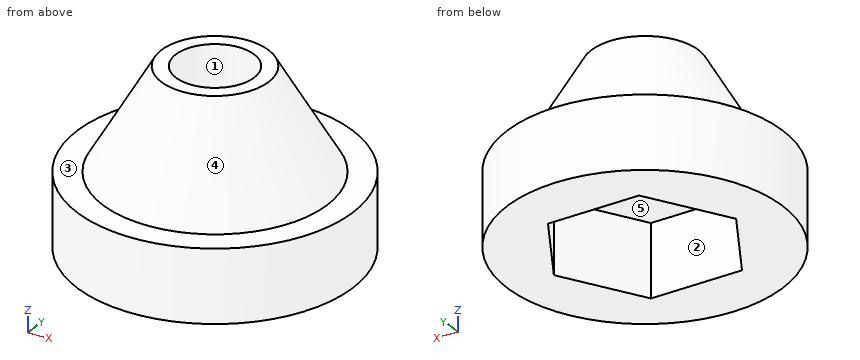
from build123d import *

# Parameters (mm, degrees)
POCKET_DEPTH = 5


with BuildPart() as part:
    # Sketch → Revolution (revolve)
    with BuildSketch(Plane.XZ):
        Polygon((2.7, 12), (2.7, 0), (9.5, 0), (9.5, 5), (7.741452, 5), (3.7, 12), align=None)
    revolve(axis=Axis((0, 0, 0), (0, 0, 1)))

    # Sketch001 (on DatumPlane) → Pocket (cut)
    with BuildSketch(Plane(origin=(0, 0, 0), x_dir=(1, 0, 0), z_dir=(0, 0, -1))):
        Polygon((3.175426, -5.5), (6.350853, 0), (3.175426, 5.5), (-3.175426, 5.5), (-6.350853, 0), (-3.175426, -5.5), align=None)
    extrude(amount=-POCKET_DEPTH, mode=Mode.SUBTRACT)


solid = part.part
For this review, take the finished solid that the model builds, in its own axes (mm). Face numbers are marked on the shaded views. A direction names the side the tool comes from. Give positions to 0.01 mm unless a question says otherwise; leave off trailing zeros. Loops run counter-clockwise (first coordinate to the right, second up) from the corner with the lowest first, then second, coordinate; pieces in that order, holes last. Notation, with made-up numbers: M -17,-25.75 L 24,-25.75 A15 cw 24,-4.75 Z; hole C -10.75,33.5 d9. An arc over 180 degrees is marked long. Put each result on its own line as item: value. Start each with the question number.
(1) Add section D-D, the plane z = 10. Write out the cut boundary in (x, y).
(2) Machinability: for the marked faces 1 and 2, which of the approach directions +Z, -Z, +X, -X, +Y, -Y give a long, thin tool a straight path to every point of the face, cutting with its end or side? Answer none if there is none.
(3) The part is to be moulded in two halves that separate along Y. For the marked faces 3, 4 and 5, say which applies: +Y half, -Y half, draft (parallel to the pull), parting line (faces both ways), or undercut.
(4) For pin 1 (2 mm diameter, centred on x = 6.5, y = 3, fed in from -Z); pin 2 (6 mm diameter, centred on y = 1.5, z = 9, fed in from +X); pin 3 (1.5 mm diameter, centred on y = -4.5, z = 2, fed in from -X); pin 4 (5 mm diameter, centred on x = 7.5, y = 0.5, fed in from +Z), all flat-tipped, find the tip position at first contact; note any pin that passes through.
(5) Wall thickness on L1, parallel to Z at x = 1.75, y = 8.25; L2, parallel to Y at x = 0, z = 2.5; L3, parallel to X at y = 0.75, z = 6: over which ranges is each line inside the solid? List them lowest first.
(6) Add section B-B, the plane z = 4.5. Write out the cut boundary in (x, y), then the cut area to 3 significant figures.
(7) Add section C-C, the plane z = 7.25. Write out the cut boundary in (x, y).
(8) Add section A-A, the plane x = 0. Write out the cut boundary in (y, z), then the cut area to 3 significant figures.
Result:
1. outline: C 0,0 d9.71; hole C 0,0 d5.4
2. face 1: +Z, -Z
2. face 2: -Z
3. face 3: draft
3. face 4: parting line
3. face 5: undercut
4. pin 1: stops at z = 0
4. pin 2: stops at x = 7.07
4. pin 3: stops at x = -8.73
4. pin 4: stops at z = 9.72
5. L1: z = 0 to 5
5. L2: y = -9.5 to -5.5, 5.5 to 9.5
5. L3: x = -7.12 to -2.59, 2.59 to 7.12
6. outline: C 0,0 d19; hole M -6.35,0 L -3.18,-5.5 L 3.18,-5.5 L 6.35,0 L 3.18,5.5 L -3.18,5.5 Z
6. area: 179 mm^2
7. outline: C 0,0 d12.88; hole C 0,0 d5.4
8. outline: M -9.5,0 L -5.5,0 L -5.5,5 L -2.7,5 L -2.7,12 L -3.7,12 L -7.74,5 L -9.5,5 Z; M 2.7,5 L 5.5,5 L 5.5,0 L 9.5,0 L 9.5,5 L 7.74,5 L 3.7,12 L 2.7,12 Z
8. area: 82.3 mm^2
